```python
from build123d import *

# Parameters (mm, degrees)
CROQUIS1_W              = 21
CROQUIS1_H              = 21
CROQUIS1_R              = 9.325
SALIENTE_EXTRUIR1_DEPTH = 20.75
CROQUIS2_W              = 5
CROQUIS2_H              = 5
SALIENTE_EXTRUIR3_DEPTH = 1
CORTAR_EXTRUIR2_DEPTH   = 18
SALIENTE_EXTRUIR7_DEPTH = 8


with BuildPart() as part:
    # Croquis1 → Saliente-Extruir1 (new, symmetric)
    with BuildSketch(Plane.XY):
        Rectangle(CROQUIS1_W, CROQUIS1_H)
        Circle(CROQUIS1_R, mode=Mode.SUBTRACT)
    extrude(amount=SALIENTE_EXTRUIR1_DEPTH, both=True)

    # Croquis2 → Saliente-Extruir3 (add)
    with BuildSketch(Plane(origin=(0, 0, -20.75), x_dir=(-1, 0, 0), z_dir=(0, 0, -1))):
        with Locations((-7.5, 7.5)):
            Rectangle(CROQUIS2_W, CROQUIS2_H)
        with Locations((7.5, 7.5)):
            Rectangle(CROQUIS2_W, CROQUIS2_H)
        with Locations((7.5, -7.5)):
            Rectangle(CROQUIS2_W, CROQUIS2_H)
        with Locations((-7.5, -7.5)):
            Rectangle(CROQUIS2_W, CROQUIS2_H)
    extrude(amount=SALIENTE_EXTRUIR3_DEPTH)

    # Croquis8 → Cortar-Extruir2 (cut)
    with BuildSketch(Plane.XY.offset(20.75)):
        Polygon((-10.55, -5.962588103), (-8.75, -5.433176338), (-8.75, -8.566823662), (-10.55, -8.037411897), align=None)
        Polygon((-10.55, 7.037411897), (-10.55, 4.962588103), (-8.75, 4.433176338), (-8.75, 7.566823662), align=None)
    extrude(amount=-CORTAR_EXTRUIR2_DEPTH, mode=Mode.SUBTRACT)

    # Croquis9 → Saliente-Extruir7 (add)
    with BuildSketch(Plane(origin=(0, 0, -20.75), x_dir=(-1, 0, 0), z_dir=(0, 0, -1))):
        Polygon((6, -10.5), (8, -10.5), (8.5, -12.2), (5.5, -12.2), align=None)
        Polygon((-4.5, -12.2), (-5, -10.5), (-7, -10.5), (-7.5, -12.2), align=None)
    extrude(amount=-SALIENTE_EXTRUIR7_DEPTH)


solid = part.part
```
Here's how the part is built. I have some questions about the finished solid (model axes, mm). A direction names the side the tool comes from. Give positions to 0.01 mm unless a question says otherwise; leave off trailing zeros. Order: outer loops, then holes, each group sorted by start corner. A loop starts at its lowest first (then second) coordinate and runs counter-clockwise, first axis right, second up. Notation, with made-up numbers: (-37, 16.5) -> (-12, 16.5) arc R10 ccw to (-12, 28.5) -> close; hole circle Ø3 at (53.5, -1). An arc over 180 degrees is marked (long way). Use CSV: the item, a comma, the result in double quotes. Start each with the question number.
Item 1: Suppose I cut it at D-D (z = -18.5). List the corners of the cut face in (x, y) for me (3 decimals).
Item 2: Suppose I cut it at A-A (x = 0). List the corners of the cut face in (y, z) for me (3 decimals).
Item 3: On a 3-axis mill with a long thin cutter (end or side, diameter ignored), from which of +Z, -Z, +X, -X, +Y, -Y can I reach the whole of each face in a straight line? I mean faces 5 (the flat face through (10, -8, -21)), 6 (the flat face through (-9.637, 4.694, 11.876)), 7 (the flat face through (8, 5, -21)), 8 (the flat face through (6, -11, -12.75)), 9 (the flat face through (4.746, -11.362, -16.806)). Say none if no direction works.
Item 4: I'm going to push flat-ended pins straight in: P1, Ø1.4, axis at x = 6, y = -11.5, coming from the +Z side; P2, Ø2, axis at x = -1, z = -3, coming from the -Y side; P3, Ø0.5, axis at x = -9.5, y = -7.5, coming from the +Z side; P4, Ø2, axis at x = 5, y = 2.5, coming from the +Z side. Where does each tip first touch, or does it pass through?
Item 5: Suppose I cut it at B-B (z = 16). List the corners of the cut face in (x, y) for me (3 decimals).
Item 6: If I drill on probe 1 along Y at (x, z) = (0, -0.5) (3 decimals); probe 2 along X at (y, z) = (3, -8); probe 3 along Y at (x, z) = (2, 6.5), over which ranges is the centre line in solid material (lowest first)? Write a range as [from, to].
Item 7: Thinking about a two-plate mould opening in X: for faces 1 (the flat face through (8, 10, -21)), 2 (the flat face through (-6, 6, -20.75)), 3 (the flat face through (-9.613, -8.313, 11.876)), 4 (the flat face through (7.246, -11.338, -16.806)), which applies, pulls with the +X half, pulls with the -X half, needs draft (parallel to the pull), parting line crosses it, or undercut?
Answer block:
1,outline,"(-10.5, -10.5) -> (-8, -10.5) -> (-8.5, -12.2) -> (-5.5, -12.2) -> (-6, -10.5) -> (5, -10.5) -> (4.5, -12.2) -> (7.5, -12.2) -> (7, -10.5) -> (10.5, -10.5) -> (10.5, 10.5) -> (-10.5, 10.5) -> close; hole circle Ø18.65 at (0, 0)"
2,outline,"(-10.5, -20.75) -> (-9.325, -20.75) -> (-9.325, 20.75) -> (-10.5, 20.75) -> close; (9.325, -20.75) -> (10.5, -20.75) -> (10.5, 20.75) -> (9.325, 20.75) -> close"
3,face 5,"-Z, +X, +Y, -Y"
3,face 6,"+Z"
3,face 7,"-Z, +X, -X"
3,face 8,"+Z, +X, -X, -Y"
3,face 9,"+Z, -Z"
4,P1,"stops at z = -12.75"
4,P2,"stops at y = -10.5"
4,P3,"stops at z = 2.75"
4,P4,"passes through"
5,outline,"(-10.5, -10.5) -> (10.5, -10.5) -> (10.5, 10.5) -> (-10.5, 10.5) -> (-10.5, 7.052) -> (-8.75, 7.567) -> (-8.75, 4.433) -> (-10.5, 4.948) -> (-10.5, -5.948) -> (-8.75, -5.433) -> (-8.75, -8.567) -> (-10.5, -8.052) -> close; hole circle Ø18.65 at (0, 0)"
6,probe 1,"y = [-10.5, -9.325], [9.325, 10.5]"
6,probe 2,"x = [-10.5, -8.83], [8.83, 10.5]"
6,probe 3,"y = [-10.5, -9.11], [9.11, 10.5]"
7,face 1,"needs draft"
7,face 2,"undercut"
7,face 3,"undercut"
7,face 4,"pulls with the +X half"
